```python
from build123d import *

# Parameters (mm, degrees)
PAD_DEPTH            = 6.5
POCKET_DEPTH         = 6
SKETCH002_R          = 13.5
POCKET001_DEPTH      = 1
SKETCH003_W          = 5.4
SKETCH003_H          = 6.5
PAD001_DEPTH         = 4.5
POCKET002_DEPTH      = 10
SKETCH010_W          = 3.95
SKETCH010_H          = 6.5
PAD002_DEPTH         = 4.5
POCKET005_DEPTH      = 10
SKETCH014_R          = 20.45
SKETCH014_R_2        = 19.5
POCKET008_DEPTH      = 0.3
SKETCH015_R          = 2.2
SKETCH015_R_2        = 0.975
PAD003_DEPTH         = 2
POCKET009_DEPTH      = 4
POCKET010_DEPTH      = 4
PAD004_DEPTH         = 4
SKETCH019_R          = 0.6
POCKET011_DEPTH      = 2
SKETCH020_R          = 0.6
POCKET012_DEPTH      = 2
POCKET013_DEPTH      = 12.151
POCKET013_DEPTH_BACK = 36.251


with BuildPart() as part:
    # Sketch → Pad (new body)
    with BuildSketch(Plane.XY):
        with BuildLine():
            Line((-22.5019915649, 16), (-22.5019915649, -16))
            Line((-22.5019915649, -16), (-16.2858834577, -17.9000000001))
            ThreePointArc((-16.2858834577, -17.9000000001), (0.2206895737, -24.1989937004), (16.6096357576, -17.5999999999))
            Line((16.6096357576, -17.5999999999), (24.9082802252, -17.45))
            Line((24.9082802252, 17.45), (24.9082802252, -17.45))
            Line((16.6096357576, 17.6), (24.9082802252, 17.45))
            ThreePointArc((16.6096357576, 17.6), (0.2206895736, 24.1989937004), (-16.2858834578, 17.9))
            Line((-22.5019915649, 16), (-16.2858834578, 17.9))
        make_face()
    extrude(amount=PAD_DEPTH)

    # Sketch001 → Pocket (cut)
    with BuildSketch(Plane.XY):
        with BuildLine():
            Line((-14.8539557021, 16.9), (-21.2122180433, 15.55))
            Line((-21.2122180433, 15.55), (-21.2122180433, -15.55))
            Line((-21.2122180433, -15.55), (-14.8539557021, -16.9))
            ThreePointArc((-14.8539557021, -16.9), (-0.0760301383, -22.4998715423), (14.739402973, -17))
            Line((14.739402973, -17), (23.6191552218, -16.4))
            Line((23.6191552218, 16.4), (23.6191552218, -16.4))
            Line((14.739402973, 17), (23.6191552218, 16.4))
            ThreePointArc((14.739402973, 17), (-0.0760301383, 22.4998715423), (-14.8539557021, 16.9))
        make_face()
    extrude(amount=POCKET_DEPTH, mode=Mode.SUBTRACT)

    # Sketch002 (on Face19 of Pocket) → Pocket001 (cut)
    with BuildSketch(Plane(origin=(0, 0, 6), x_dir=(1, 0, 0), z_dir=(0, 0, -1))):
        Circle(SKETCH002_R)
    extrude(amount=-POCKET001_DEPTH, mode=Mode.SUBTRACT)

    # Sketch003 (on Face7 of Pad) → Pad001 (join)
    with BuildSketch(Plane.YZ.offset(24.9082802252)):
        with Locations((-14.75, 3.25)):
            Rectangle(SKETCH003_W, SKETCH003_H)
        with Locations((14.75, 3.25)):
            Rectangle(SKETCH003_W, SKETCH003_H)
    extrude(amount=PAD001_DEPTH)

    # Sketch006 (on Face22 of Pad001) → Pocket002 (cut)
    with BuildSketch(Plane.XY.offset(6.5)):
        with BuildLine():
            ThreePointArc((24.9082802252, 17.45), (26.9423471239, 15.7065020586), (29.4082802252, 14.6594169811))
            Line((29.4082802252, 17.45), (29.4082802252, 14.6594169811))
            Line((29.4082802252, 17.45), (24.9082802252, 17.45))
        make_face()
        with BuildLine():
            ThreePointArc((29.4082802252, -14.6594169811), (26.9423471239, -15.7065020586), (24.9082802252, -17.45))
            Line((29.4082802252, -17.45), (24.9082802252, -17.45))
            Line((29.4082802252, -14.6594169811), (29.4082802252, -17.45))
        make_face()
    extrude(amount=-POCKET002_DEPTH, mode=Mode.SUBTRACT)

    # Sketch010 (on Face3 of Pad) → Pad002 (join)
    with BuildSketch(Plane(origin=(-22.5019915649, 0, 0), x_dir=(0, -1, 0), z_dir=(-1, 0, 0))):
        with Locations((-14.025, 3.25)):
            Rectangle(SKETCH010_W, SKETCH010_H)
        with Locations((14.025, 3.25)):
            Rectangle(SKETCH010_W, SKETCH010_H)
    extrude(amount=PAD002_DEPTH)

    # Sketch011 (on Face28 of Pad002) → Pocket005 (cut)
    with BuildSketch(Plane.XY.offset(6.5)):
        Polygon((-27.0019915649, 16), (-22.5019915649, 16), (-27.0019915649, 14.5), align=None)
        Polygon((-22.5019915649, -16), (-27.0019915649, -14.5), (-27.0019915649, -16), align=None)
    extrude(amount=-POCKET005_DEPTH, mode=Mode.SUBTRACT)

    # Sketch014 (on Face10 of Pad) → Pocket008 (cut)
    with BuildSketch(Plane.XY.offset(6.5)):
        Circle(SKETCH014_R)
        Circle(SKETCH014_R_2, mode=Mode.SUBTRACT)
    extrude(amount=-POCKET008_DEPTH, mode=Mode.SUBTRACT)

    # Sketch015 (on Face19 of Pocket) → Pad003 (join)
    with BuildSketch(Plane(origin=(0, 0, 6), x_dir=(1, 0, 0), z_dir=(0, 0, -1))):
        with Locations((-18.42, 13.32)):
            Circle(SKETCH015_R)
        with Locations((-18.42, 13.32)):
            Circle(SKETCH015_R_2, mode=Mode.SUBTRACT)
        with Locations((7.27, 18.56)):
            Circle(SKETCH015_R)
        with Locations((7.27, 18.56)):
            Circle(SKETCH015_R_2, mode=Mode.SUBTRACT)
        with Locations((5.37, -19.79)):
            Circle(SKETCH015_R)
        with Locations((5.37, -19.79)):
            Circle(SKETCH015_R_2, mode=Mode.SUBTRACT)
        with Locations((-18.42, -13.32)):
            Circle(SKETCH015_R)
        with Locations((-18.42, -13.32)):
            Circle(SKETCH015_R_2, mode=Mode.SUBTRACT)
    extrude(amount=PAD003_DEPTH)

    # Sketch016 → Pocket009 (cut)
    with BuildSketch(Plane(origin=(0, 0, 0), x_dir=(-1, 0, 0), z_dir=(0, 0, 1))):
        with BuildLine():
            Line((-5, 23.6778377391), (-5, 21.9374109685))
            ThreePointArc((5, 21.9374109685), (0, 22.5), (-5, 21.9374109685))
            Line((5, 23.6778377391), (5, 21.9374109685))
            ThreePointArc((5, 23.6778377391), (0, 24.2), (-5, 23.6778377391))
        make_face()
    extrude(amount=POCKET009_DEPTH, mode=Mode.SUBTRACT)

    # Sketch017 → Pocket010 (cut)
    with BuildSketch(Plane(origin=(0, 0, 0), x_dir=(-1, 0, 0), z_dir=(0, 0, 1))):
        with BuildLine():
            Line((-3.499984119, -22.2261132717), (-3.5, -23.9455632634))
            ThreePointArc((-3.5, -23.9455632634), (0, -24.2000019575), (3.5, -23.9455632634))
            Line((3.5000158811, -22.2261082701), (3.5, -23.9455632634))
            ThreePointArc((-3.499984119, -22.2261132717), (1.60767e-05, -22.5), (3.5000158811, -22.2261082701))
        make_face()
        with BuildLine():
            ThreePointArc((-13.9498796389, -17.6536358312), (-11.25, -19.4855715851), (-8.3135572795, -20.9077680626))
            Line((-8.3135572795, -20.9077680626), (-8.9416927184, -22.487466094))
            ThreePointArc((-15.0038705449, -18.987466094), (-12.1, -20.9578147716), (-8.9416927184, -22.487466094))
            Line((-13.9498796389, -17.6536358312), (-15.0038705449, -18.987466094))
        make_face()
        with BuildLine():
            ThreePointArc((8.3135572795, -20.9077680626), (11.25, -19.4855715851), (13.9498796389, -17.6536358312))
            Line((13.9498796389, -17.6536358312), (15.0038705449, -18.987466094))
            ThreePointArc((8.9416927184, -22.487466094), (12.1, -20.9578147716), (15.0038705449, -18.987466094))
            Line((8.3135572795, -20.9077680626), (8.9416927184, -22.487466094))
        make_face()
    extrude(amount=POCKET010_DEPTH, mode=Mode.SUBTRACT)

    # Sketch018 (on Face8 of Pocket005) → Pad004 (join)
    with BuildSketch(Plane(origin=(0, 0, 0), x_dir=(1, 0, 0), z_dir=(0, 0, -1))):
        Polygon((-27.0019915649, 14.5), (-27.0019915649, 12.05), (-22.5019915649, 12.05), (-22.5019915649, 16), align=None)
        Polygon((-27.0019915649, -12.05), (-22.5019915649, -12.05), (-22.5019915649, -16), (-27.0019915649, -14.5), align=None)
        with BuildLine():
            Line((24.9082802252, 17.45), (24.9082802252, 12.05))
            Line((29.4082802252, 12.05), (24.9082802252, 12.05))
            Line((29.4082802252, 14.6594169811), (29.4082802252, 12.05))
            ThreePointArc((24.9082802252, 17.45), (26.9423471239, 15.7065020586), (29.4082802252, 14.6594169811))
        make_face()
        with BuildLine():
            Line((24.9082802252, -12.05), (24.9082802252, -17.45))
            ThreePointArc((29.4082802252, -14.6594169811), (26.9423471239, -15.7065020586), (24.9082802252, -17.45))
            Line((29.4082802252, -12.05), (29.4082802252, -14.6594169811))
            Line((24.9082802252, -12.05), (29.4082802252, -12.05))
        make_face()
    extrude(amount=PAD004_DEPTH)

    # Sketch019 (on Face64 of Pad004) → Pocket011 (cut)
    with BuildSketch(Plane.XZ.offset(-12.05)):
        with Locations((28.1082802252, -2.7)):
            Circle(SKETCH019_R)
        with Locations((-25.7019915649, -2.7)):
            Circle(SKETCH019_R)
    extrude(amount=-POCKET011_DEPTH, mode=Mode.SUBTRACT)

    # Sketch020 (on Face50 of Pocket011) → Pocket012 (cut)
    with BuildSketch(Plane(origin=(0, -12.05, 0), x_dir=(-1, 0, 0), z_dir=(0, 1, 0))):
        with Locations((-28.1082802252, -2.7)):
            Circle(SKETCH020_R)
        with Locations((25.7019915649, -2.7)):
            Circle(SKETCH020_R)
    extrude(amount=-POCKET012_DEPTH, mode=Mode.SUBTRACT)

    # Sketch021 (on Face48 of Pocket012) → Pocket013 (cut, two sides)
    with BuildSketch(Plane.XZ.offset(-12.05)) as pocket013_sk:
        with BuildLine():
            ThreePointArc((29.4082802252, 0), (28.1735037783, 3.9528470752), (24.9082802252, 6.5))
            Line((24.9082802252, 6.5), (29.4082802252, 6.5))
            Line((29.4082802252, 6.5), (29.4082802252, 0))
        make_face()
        with BuildLine():
            ThreePointArc((24.9082802252, -1.478433716), (25.9291187082, -3.0916708473), (27.6082802252, -4))
            Line((24.9082802252, -4), (27.6082802252, -4))
            Line((24.9082802252, -1.478433716), (24.9082802252, -4))
        make_face()
    extrude(amount=-POCKET013_DEPTH, mode=Mode.SUBTRACT)
    extrude(pocket013_sk.sketch, amount=POCKET013_DEPTH_BACK, mode=Mode.SUBTRACT)


solid = part.part
```
Input: part model. Units: mm. Frame: model coordinates. A direction names the side the tool comes from. Give positions to 0.01 mm unless a question says otherwise; leave off trailing zeros. Order: outer loops, then holes, each group sorted by start corner. A loop starts at its lowest first (then second) coordinate and runs counter-clockwise, first axis right, second up. Notation, with made-up numbers: (41.5, 2.5) - (93.5, 2.5) arc R30 ccw to (93.5, 40.5) - close; hole circle Ø2 at (-35, 54.5). An arc over 180 degrees is marked (long way). Use a Markdown table: item, result.
(1) Section query B-B (x = -2). Output: boundary loops of the cut face in (y, z), then the cut area to 3 significant figures.
Computed values:
| item | result |
|---|---|
| outline | (-24.12, 4) - (-22.41, 4) - (-22.41, 6) - (-13.35, 6) - (-13.35, 6.5) - (-19.4, 6.5) - (-19.4, 6.2) - (-20.35, 6.2) - (-20.35, 6.5) - (-24.12, 6.5) - close; (13.35, 6) - (22.41, 6) - (22.41, 4) - (24.12, 4) - (24.12, 6.5) - (20.35, 6.5) - (20.35, 6.2) - (19.4, 6.2) - (19.4, 6.5) - (13.35, 6.5) - close |
| area | 17.0 mm2 |
(2) Draft query along Z for faces 1 (the flat face through (7, -20, 4)), 2 (the flat face through (29.408, -13, -2)), 3 (the cylindrical face through (-25.148, 13.036, -2.93)). Return one class per face: released by +Z, released by -Z, zero draft, split by the parting line, or undercut.
Computed values:
| item | result |
|---|---|
| face 1 | released by -Z |
| face 2 | zero draft |
| face 3 | undercut |
(3) Line query: line 1 (Y direction, x = 0, z = 6.35); line 2 (Y direction, x = -18.42, z = 4.45) (3 decimals); line 3 (X direction, y = 12, z = 5.5). Output: solid intervals per line, ascending. Write a range as from..to.
Computed values:
| item | result |
|---|---|
| line 1 | y = -24.2..-20.45, -19.5..-13.5, 13.5..19.5, 20.45..24.2 |
| line 2 | y = -17.248..-16.143, -15.52..-14.295, -12.345..-11.12, 11.12..12.345, 14.295..15.52, 16.143..17.248 |
| line 3 | x = -22.5..-21.21, -20.18..-16.66, 23.62..24.91 |
(4) Section query C-C (y = -18.56). Output: boundary loops of the cut face in (x, z) (3 decimals).
Computed values:
| item | result |
|---|---|
| outline | (-15.53, 0) - (-12.719, 0) - (-12.719, 6) - (5.07, 6) - (5.07, 4) - (6.295, 4) - (6.295, 6) - (8.245, 6) - (8.245, 4) - (9.47, 4) - (9.47, 6) - (12.719, 6) - (12.719, 0) - (15.53, 0) - (15.53, 6.5) - (8.587, 6.5) - (8.587, 6.2) - (5.981, 6.2) - (5.981, 6.5) - (-5.981, 6.5) - (-5.981, 6.2) - (-8.587, 6.2) - (-8.587, 6.5) - (-15.53, 6.5) - close |
(5) Pin query (flat end, axial travel): pin 1 (1.3 mm diameter, centred on x = 27.5, z = 3, fed in from +Y); pin 2 (4 mm diameter, centred on y = 14, z = 3.5, fed in from +X); pin 3 (3.5 mm diameter, centred on x = -17.5, y = 14, fed in from -Z); pin 4 (2 mm diameter, centred on y = -19, z = -1.5, fed in from +X). Return the tip coordinate at first contact, or that it passes through.
Computed values:
| item | result |
|---|---|
| pin 1 | stops at y = 15.76 |
| pin 2 | stops at x = 29.24 |
| pin 3 | stops at z = 4 |
| pin 4 | passes through |
(6) Section query A-A (z = -0.75). Output: boundary loops of the cut face in (x, y).
Computed values:
| item | result |
|---|---|
| outline | (-27, -14.5) - (-22.5, -16) - (-22.5, -12.05) - (-27, -12.05) - close; (-27, 12.05) - (-22.5, 12.05) - (-22.5, 16) - (-27, 14.5) - close; (24.91, -17.45) arc R8.76 cw to (29.41, -14.66) - (29.41, -12.05) - (24.91, -12.05) - close; (24.91, 12.05) - (29.41, 12.05) - (29.41, 14.66) arc R8.76 cw to (24.91, 17.45) - close |
(7) Access query for faces 4 (the flat face through (23.619, 0, 3)), 5 (the flat face through (27, -12.05, 1)), 6 (the cylindrical face through (-25.1, -13, -2.7)). Directions: +Z, -Z, +X, -X, +Y, -Y. A direction counts if a zero-diameter tool reaches every point of the face in a straight line with its end or side. Return the directions, or none.
Computed values:
| item | result |
|---|---|
| face 4 | -Z |
| face 5 | +Z, -Z, +X |
| face 6 | none |
